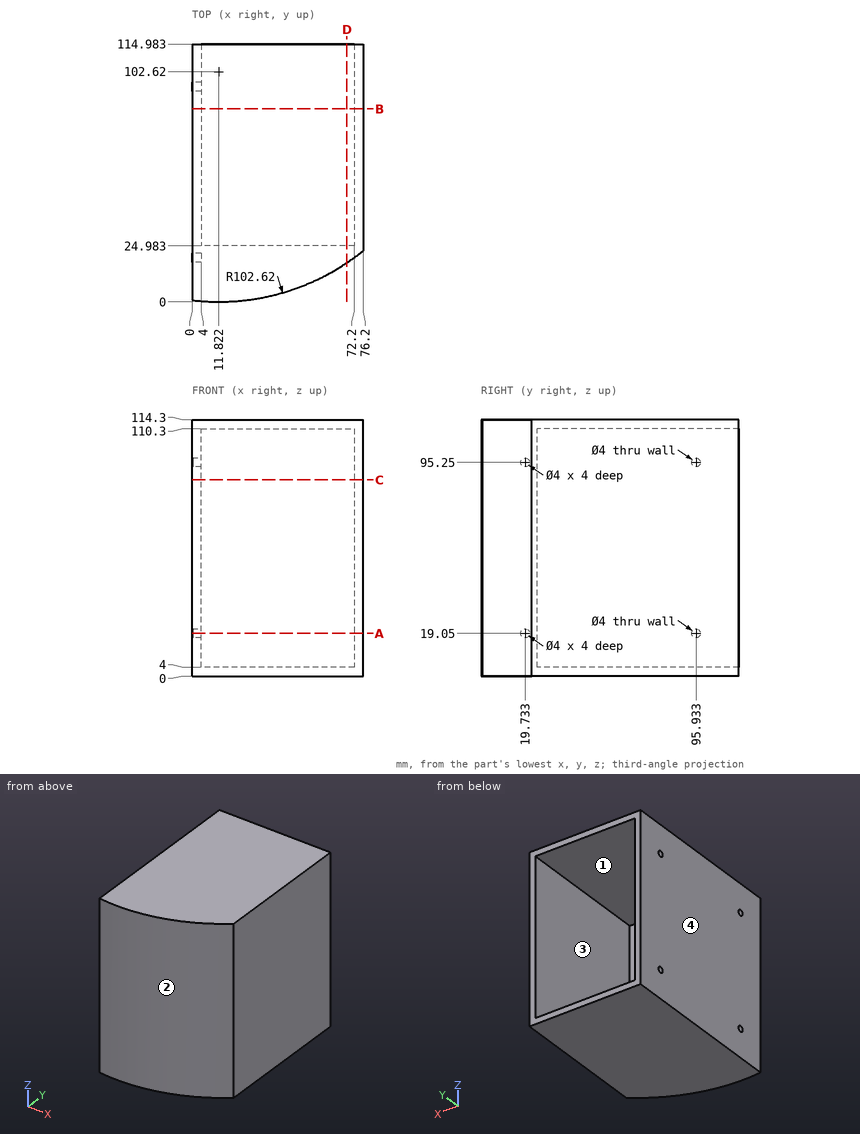
Check sheet for the drawn part. Datum: minimum x, y, z corner. Units: mm. Coordinates: 2 decimals unless noted, no trailing zeros. Loops run counter-clockwise (first coordinate to the right, second up) from the corner with the lowest first, then second, coordinate; pieces in that order, holes last. Notation, with made-up numbers: (56, 20.25) -> (88, 20.25) arc R26 cw to (88, 44.25) -> close; hole circle Ø3 at (16, 42.25). An arc over 180 degrees is marked (long way). Write each question's results on one line, items separated by ' | '.
Item 1: Material ranges on L1, parallel to Z at x = 16, y = 44.5; L2, parallel to X at y = 102.5, z = 26.5; L3, parallel to Y at x = 13, z = 97, recorded low to high.
Found:
L1: z = 0 to 4, 110.3 to 114.3 | L2: x = 0 to 4, 72.2 to 76.2 | L3: y = 0.01 to 24.98
Item 2: Section check D-D, the plane x = 69. Enter the section's corners in (y, z) (1 decimal).
Found:
outline: (17.4, 0) -> (115, 0) -> (115, 4) -> (25, 4) -> (25, 110.3) -> (115, 110.3) -> (115, 114.3) -> (17.4, 114.3) -> close
Item 3: Section check C-C, the plane z = 87.5. Enter the section's corners in (x, y) (1 decimal), plus the area to 3 significant figures.
Found:
outline: (0, 0.7) arc R102.6 ccw to (76.2, 22.7) -> (76.2, 115) -> (72.2, 115) -> (72.2, 25) -> (4, 25) -> (4, 115) -> (0, 115) -> close | area: 2,160 mm2
Item 4: Mould release check, pull along X, two halves, no side actions. Record for the marked faces 1, 2, 3 and 4: +X half, -X half, draft (parallel to the pull), parting line (faces both ways), or undercut.
Found:
face 1: undercut | face 2: parting line | face 3: undercut | face 4: -X half
Item 5: Gauge pin test, flat ends, axial feed: pin 1 (6 mm diameter, centred on x = 9, y = 72.5, fed in from -Z); pin 2 (2.5 mm diameter, centred on y = 19.73, z = 95.25, fed in from -X); pin 3 (1 mm diameter, centred on x = 10, z = 67.5, fed in from -Y); pin 4 (1.5 mm diameter, centred on x = 17.5, z = 35.5, fed in from -Y). Record the tip position at first contact, or that the pin passes through.
Found:
pin 1: stops at z = 0 | pin 2: stops at x = 4 | pin 3: stops at y = 0.01 | pin 4: stops at y = 0.12
Item 6: Section check A-A, the plane z = 19.05. Enter the section's corners in (x, y) (1 decimal).
Found:
outline: (0, 0.7) arc R102.6 ccw to (76.2, 22.7) -> (76.2, 115) -> (72.2, 115) -> (72.2, 25) -> (4, 25) -> (4, 93.9) -> (0, 93.9) -> (0, 21.7) -> (4, 21.7) -> (4, 17.7) -> (0, 17.7) -> close; (0, 97.9) -> (4, 97.9) -> (4, 115) -> (0, 115) -> close
Item 7: Section check B-B, the plane y = 86. Enter the section's corners in (x, z).
Found:
outline: (0, 0) -> (76.2, 0) -> (76.2, 114.3) -> (0, 114.3) -> close; hole (4, 4) -> (72.2, 4) -> (72.2, 110.3) -> (4, 110.3) -> close
